Source: CAD feature listing. Evaluate the final solid. Frame: model axes, mm. Face numbers are marked on the shaded views. A direction names the side the tool comes from. Coordinates: 2 decimals unless noted, no trailing zeros. Loops run counter-clockwise (first coordinate to the right, second up) from the corner with the lowest first, then second, coordinate; pieces in that order, holes last. Notation, with made-up numbers: M 49.25,20.25 L 68.25,20.25 A9 ccw 68.25,34.25 Z; hole C -11,75 d8. An arc over 180 degrees is marked long. Write each question's results on one line, items separated by ' | '. Start each with the question number.
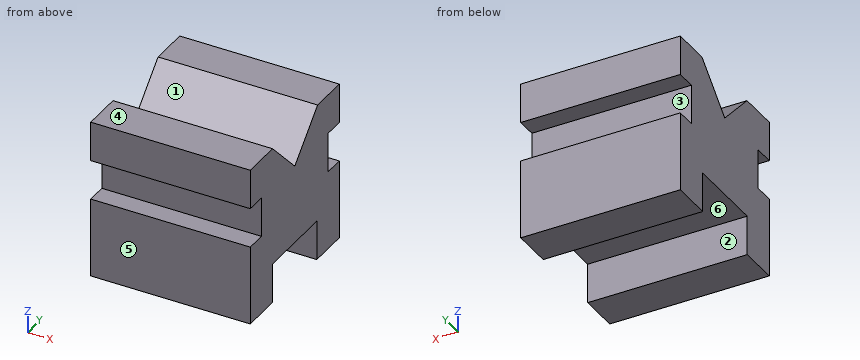
from build123d import *

# Parameters (mm, degrees)
F0_W     = 101.6
F0_H     = 101.6
F1_DEPTH = 101.6
F2_W     = 12.7
F2_H     = 25.4
F2_W_2   = 25.644753
F2_W_3   = 25.155247
F3_DEPTH = 101.6


with BuildPart() as f1:
    # F0 (on Top) → F1 (new body)
    with BuildSketch(Plane.XY):
        with Locations((-50.8, -50.8)):
            Rectangle(F0_W, F0_H)
    extrude(amount=F1_DEPTH)

    # F2 (on face) → F3 (cut)
    with BuildSketch(Plane.YZ):
        Polygon((-50.8, 101.6), (-76.2, 101.6), (-50.8, 75.85644), align=None)
        Polygon((-50.8, 101.6), (-50.8, 75.85644), (-24.708233, 101.6), align=None)
        with Locations((-95.25, 63.5)):
            Rectangle(F2_W, F2_H)
        with Locations((-63.622376, 12.7)):
            Rectangle(F2_W_2, F2_H)
        with Locations((-38.222376, 12.7)):
            Rectangle(F2_W_3, F2_H)
        with Locations((-6.35, 63.5)):
            Rectangle(F2_W, F2_H)
    extrude(amount=-F3_DEPTH, mode=Mode.SUBTRACT)


solid = f1.part
Item 1: Mould query, pull axis Y, two halves, no side actions, for the marked faces 4, 5 and 6. Classes: +Y half, -Y half, draft (parallel to the pull), parting line (faces both ways), or undercut.
Item 2: Access query for the marked faces 1, 2 and 3. Directions: +Z, -Z, +X, -X, +Y, -Y. A direction counts if a zero-diameter tool reaches every point of the face in a straight line with its end or side. Return the directions, or none.
Item 3: Cut plane A-A (z = 88). Output: boundary loops of the cut face in (x, y).
Item 4: Cut plane B-B (y = -8). Output: boundary loops of the cut face in (x, z).
Item 5: Line query: probe 1 along Y at (x, z) = (-47, 20); probe 2 along Z at (x, y) = (-71.5, -92.5); probe 3 along Y at (x, z) = (-27, 51). Output: solid intervals per line, ascending.
Item 6: Cut plane C-C (x = -20). Output: boundary loops of the cut face in (y, z).
Item 7: Cut plane D-D (z = 55). Output: boundary loops of the cut face in (x, y), then the cut area to 3 significant figures.
Item 8: First-contact query: pin 1 Ø2 at (x, y) = (-78.5, -27.5) entering from +Z; pin 2 Ø12.5 at (x, z) = (-65.5, 68.5) entering from -Y; pin 3 Ø12 at (x, y) = (-60, -48.5) entering from -Z. Flat tips, straight axial feed; report the tip coordinate or a pass-through.
Response values:
1) face 4: draft | face 5: -Y half | face 6: undercut
2) face 1: +Z, +X, -X | face 2: -Z, +X, -X | face 3: +X, -X, +Y
3) outline: M -101.6,-101.6 L 0,-101.6 L 0,-62.78 L -101.6,-62.78 Z; M -101.6,-38.49 L 0,-38.49 L 0,0 L -101.6,0 Z
4) outline: M -101.6,0 L 0,0 L 0,50.8 L -101.6,50.8 Z; M -101.6,76.2 L 0,76.2 L 0,101.6 L -101.6,101.6 Z
5) probe 1: y = -101.6 to -76.44, -25.64 to 0 | probe 2: z = 0 to 50.8, 76.2 to 101.6 | probe 3: y = -88.9 to -12.7
6) outline: M -101.6,0 L -76.44,0 L -76.44,25.4 L -25.64,25.4 L -25.64,0 L 0,0 L 0,50.8 L -12.7,50.8 L -12.7,76.2 L 0,76.2 L 0,101.6 L -24.71,101.6 L -50.8,75.86 L -76.2,101.6 L -101.6,101.6 L -101.6,76.2 L -88.9,76.2 L -88.9,50.8 L -101.6,50.8 Z
7) outline: M -101.6,-88.9 L 0,-88.9 L 0,-12.7 L -101.6,-12.7 Z | area: 7,740 mm2
8) pin 1: stops at z = 99.83 | pin 2: stops at y = -88.9 | pin 3: stops at z = 25.4
